Input: part model. Units: mm. Frame: model coordinates. Face numbers are marked on the shaded views. Round coordinates to 2 decimals unless told otherwise and drop trailing zeros. Answer as a JSON object with one key per item and string values.
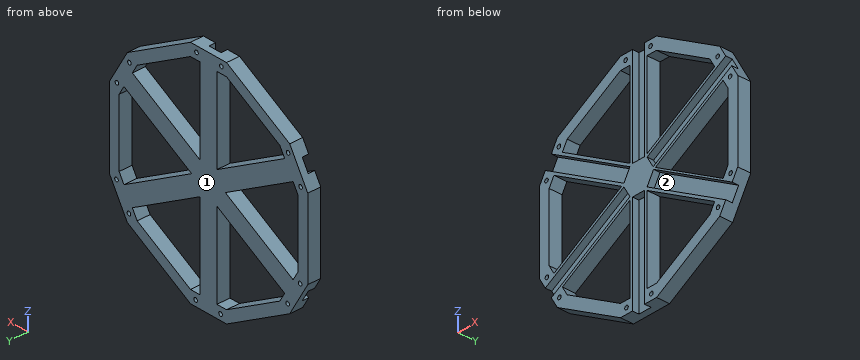
```python
from build123d import *

# Parameters (mm, degrees)
F1_DEPTH = 10
F2_W     = 10
F2_H     = 75.4743308471
F2_H_2   = 22.4482722858
F3_DEPTH = 5
F4_R     = 1.5
F5_DEPTH = 25


with BuildPart() as f1:
    # F0 (on Front) → F1 (new body)
    with BuildSketch(Plane.XZ):
        Polygon((15, 86.6025403784), (-15, 86.6025403784), (-15, 77.153906079), (-7, 77.153906079), (-7, 12.124355653), (-63.3172426656, 44.639130866), (-59.3172426656, 51.5673340962), (-67.5, 56.291651246), (-82.5, 30.3108891325), (-74.3172426656, 25.5865719827), (-70.3172426656, 32.514775213), (-14, 0), (-70.3172426656, -32.514775213), (-74.3172426656, -25.5865719827), (-82.5, -30.3108891325), (-67.5, -56.291651246), (-59.3172426656, -51.5673340962), (-63.3172426656, -44.639130866), (-7, -12.124355653), (-7, -77.153906079), (-15, -77.153906079), (-15, -86.6025403784), (15, -86.6025403784), (15, -77.153906079), (7, -77.153906079), (7, -12.124355653), (63.3172426656, -44.639130866), (59.3172426656, -51.5673340962), (67.5, -56.291651246), (82.5, -30.3108891325), (74.3172426656, -25.5865719827), (70.3172426656, -32.514775213), (14, 0), (70.3172426656, 32.514775213), (74.3172426656, 25.5865719827), (82.5, 30.3108891325), (67.5, 56.291651246), (59.3172426656, 51.5673340962), (63.3172426656, 44.639130866), (7, 12.124355653), (7, 77.153906079), (15, 77.153906079), align=None)
        Polygon((-59.3172426656, -51.5673340962), (-67.5, -56.291651246), (-15, -86.6025403784), (-15, -77.153906079), align=None)
        Polygon((-74.3172426656, 25.5865719827), (-82.5, 30.3108891325), (-82.5, -30.3108891325), (-74.3172426656, -25.5865719827), align=None)
        Polygon((-15, 77.153906079), (-15, 86.6025403784), (-67.5, 56.291651246), (-59.3172426656, 51.5673340962), align=None)
        Polygon((67.5, 56.291651246), (15, 86.6025403784), (15, 77.153906079), (59.3172426656, 51.5673340962), align=None)
        Polygon((82.5, -30.3108891325), (82.5, 30.3108891325), (74.3172426656, 25.5865719827), (74.3172426656, -25.5865719827), align=None)
        Polygon((15, -86.6025403784), (67.5, -56.291651246), (59.3172426656, -51.5673340962), (15, -77.153906079), align=None)
    extrude(amount=F1_DEPTH)

    # F2 (on face) → F3 (cut)
    with BuildSketch(Plane.XZ.offset(10)):
        Polygon((-77.5, 38.9711431703), (-72.5, 47.6313972081), (-109.8431605698, 69.1914810155), (-114.8431605698, 60.5312269776), align=None)
        with Locations((0, 48.8653749549)):
            Rectangle(F2_W, F2_H)
        Polygon((121.6227966993, 75.9924571058), (72.5, 47.6313972081), (77.5, 38.9711431703), (126.6227966993, 67.332203068), align=None)
        Polygon((77.8658404617, -38.3374889031), (72.5, -47.6313972081), (106.878233392, -67.4796795113), (112.2440738537, -58.1857712063), align=None)
        with Locations((0, -97.8266765213)):
            Rectangle(F2_W, F2_H_2)
        Polygon((-72.5, -47.6313972081), (-77.5, -38.9711431703), (-141.8294904827, -76.1117918173), (-136.8294904827, -84.7720458552), align=None)
        with Locations((0, -48.8653749549)):
            Rectangle(F2_W, F2_H)
        Polygon((-7.1373121527, -9.8942317846), (-12.1373121527, -1.2339777467), (-77.5, -38.9711431703), (-72.5, -47.6313972081), align=None)
        Polygon((-12.1373121527, 1.2339777467), (-7.1373121527, 9.8942317846), (-72.5, 47.6313972081), (-77.5, 38.9711431703), align=None)
        Polygon((72.5, 47.6313972081), (7.1373121527, 9.8942317846), (12.1373121527, 1.2339777467), (77.5, 38.9711431703), align=None)
        Polygon((12.5031526145, -0.6003234796), (7.1373121527, -9.8942317846), (72.5, -47.6313972081), (77.8658404617, -38.3374889031), align=None)
    extrude(amount=-F3_DEPTH, mode=Mode.SUBTRACT)

    # F4 (on face) → F5 (cut)
    with BuildSketch(Plane.XZ.offset(10)):
        with Locations((66.1473696845, -49.7372070773)):
            Circle(F4_R)
        with Locations((76.5132101462, -31.7830447345)):
            Circle(F4_R)
        with Locations((76.1473696845, 32.4166990016)):
            Circle(F4_R)
        with Locations((65.7815292228, 50.3708613445)):
            Circle(F4_R)
        with Locations((10, 82.153906079)):
            Circle(F4_R)
        with Locations((-10.7316809234, 82.153906079)):
            Circle(F4_R)
        with Locations((-66.1473696845, 49.7372070773)):
            Circle(F4_R)
        with Locations((-76.5132101462, 31.7830447345)):
            Circle(F4_R)
        with Locations((-76.1473696845, -32.4166990016)):
            Circle(F4_R)
        with Locations((-65.7815292228, -50.3708613445)):
            Circle(F4_R)
        with Locations((-10, -82.153906079)):
            Circle(F4_R)
        with Locations((10.7316809234, -82.153906079)):
            Circle(F4_R)
    extrude(amount=-F5_DEPTH, mode=Mode.SUBTRACT)


solid = f1.part
```
1) Draft query along Z for the marked faces 1 and 2. Return one class per face: +Z half, -Z half, draft (parallel to the pull), parting line (faces both ways), or undercut.
Output:
{"face 1": "draft", "face 2": "undercut"}
2) Section A-A, the plane y = -8. Count the separate pieces of the cut face and the enclosed holes in it, plus the area to 3 significant figures.
Output:
{"separate pieces": "1", "enclosed holes": "18", "area": "5,750 mm^2"}
3) Contact query for flat-ended pins moving along their axis: P1, Ø4, axis at y = -8.5, z = 35, coming from the +X side; P2, Ø2.5, axis at x = 10, z = 82.15, coming from the +Y side; P3, Ø8, axis at x = -0.5, z = 65, coming from the -Y side; P4, Ø5, axis at x = -10.73, z = 82.15, coming from the +Y side. Output: stop coordinate, or through.
Output:
{"P1": "stops at x = 80.95", "P2": "passes through", "P3": "stops at y = -5", "P4": "stops at y = 0"}
4) Ray query, probe 1 along Z at (x, y) = (71, -6.5); probe 2 along Z at (x, y) = (41, -0.5); probe 3 along Z at (x, y) = (-49.5, -8.25). Return the intervals inside material, ascending.
Output:
{"probe 1": "z = -50.23 to -46.77, -34.37 to -31.33, 31.33 to 35.22, 46.77 to 50.23", "probe 2": "z = -71.59 to -62.14, -31.75 to -15.59, 15.59 to 31.75, 62.14 to 71.59", "probe 3": "z = -66.68 to -57.24, -36.66 to -34.35, -22.81 to -20.5, 20.5 to 22.81, 34.35 to 36.66, 57.24 to 66.68"}
